Geometry check sheet. Reference: drawing and pictorial views, mm from the part's lowest x, y, z. A direction names the side the tool comes from. Coordinates: 2 decimals unless noted, no trailing zeros. Loops run counter-clockwise (first coordinate to the right, second up) from the corner with the lowest first, then second, coordinate; pieces in that order, holes last. Notation, with made-up numbers: (65.5, 56) -> (70.5, 56) arc R23 ccw to (70.5, 73) -> close; hole circle Ø10 at (46, 45.5). An arc over 180 degrees is marked (long way). Use CSV: the item, a comma, the result in double quotes.
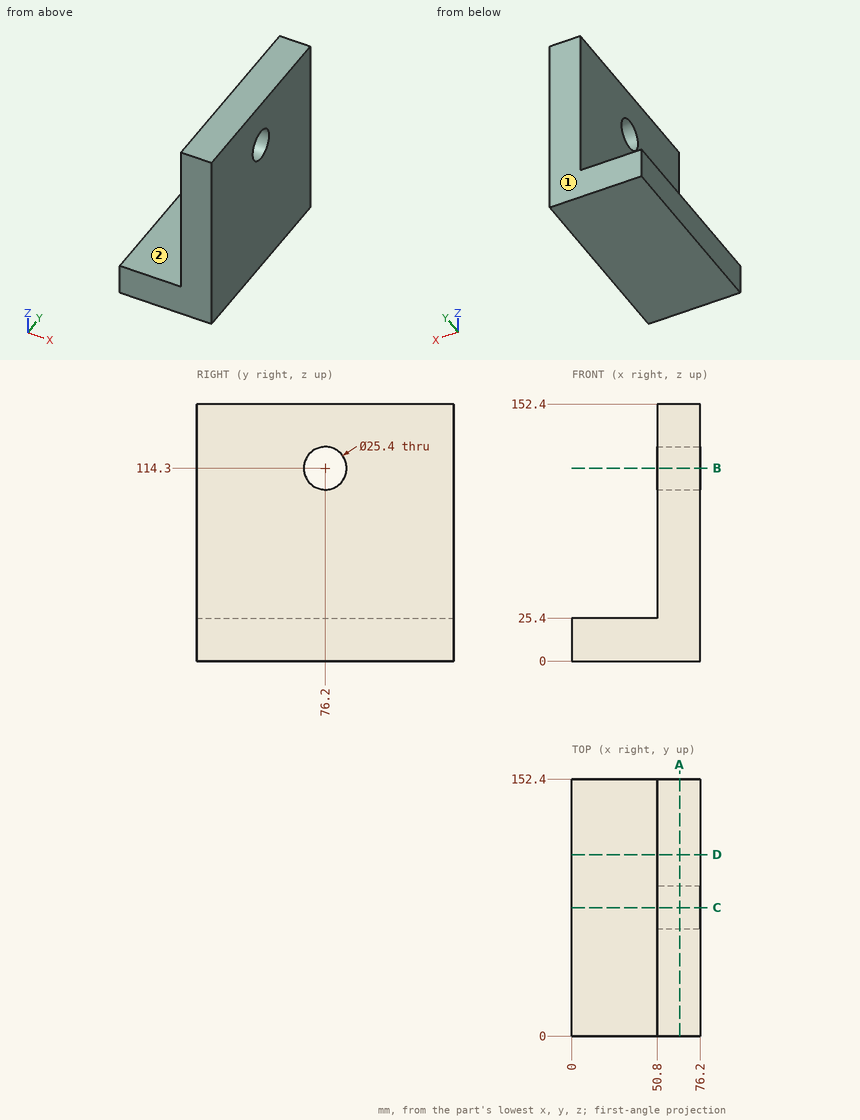
1) Go/stop test with flat-tipped pins: pin 1 Ø4 at (x, y) = (35.5, 70) entering from +Z; pin 2 Ø4 at (x, z) = (53, 136.5) entering from -Y; pin 3 Ø4 at (y, z) = (47, 58) entering from -X. Record where each tip stops, or that it passes through.
Answer below:
pin 1,"stops at z = 25.4"
pin 2,"stops at y = 0"
pin 3,"stops at x = 50.8"
2) Cross-section at D-D on y = 107.5. Record the boundary of the cut face in (x, z), and give its area (3 significant figures).
Answer below:
outline,"(0, 0) -> (76.2, 0) -> (76.2, 152.4) -> (50.8, 152.4) -> (50.8, 25.4) -> (0, 25.4) -> close"
area,"5,160 mm²"
3) Thickness scan on line 1 along Z through (x, y) = (64.5, 76.2); line 2 along Y through (x, z) = (57, 114); line 3 along X through (y, z) = (86, 45). Record the ranges inside material, lowest first. Write a range as from..to.
Answer below:
line 1,"z = 0..101.6, 127..152.4"
line 2,"y = 0..63.5, 88.9..152.4"
line 3,"x = 50.8..76.2"
4) Access from +Z, -Z, +X, -X, +Y, -Y to the whole of each face (thin tool, end or side, straight path). Record for the marked faces 1 and 2.
Answer below:
face 1,"+Z, -Z, +X, -X, +Y"
face 2,"+Z, -X, +Y, -Y"
5) Cross-section at A-A on x = 64. Record the boundary of the cut face in (y, z), and give its area (3 significant figures).
Answer below:
outline,"(0, 0) -> (152.4, 0) -> (152.4, 152.4) -> (0, 152.4) -> close; hole circle Ø25.4 at (76.2, 114.3)"
area,"22,700 mm²"
6) Cross-section at C-C on y = 76.2. Record the boundary of the cut face in (x, z), and give its area (3 significant figures).
Answer below:
outline,"(0, 0) -> (76.2, 0) -> (76.2, 101.6) -> (50.8, 101.6) -> (50.8, 25.4) -> (0, 25.4) -> close; (50.8, 127) -> (76.2, 127) -> (76.2, 152.4) -> (50.8, 152.4) -> close"
area,"4,520 mm²"
7) Cross-section at B-B on z = 114.3. Record the boundary of the cut face in (x, y).
Answer below:
outline,"(50.8, 0) -> (76.2, 0) -> (76.2, 63.5) -> (50.8, 63.5) -> close; (50.8, 88.9) -> (76.2, 88.9) -> (76.2, 152.4) -> (50.8, 152.4) -> close"
